Autodesk Inventor part; units mm, degrees
ref_plane "YZ Plane" through (0, 0, 0) normal (1, 0, 0) x (0, 1, 0)
ref_plane "XZ Plane" through (0, 0, 0) normal (0, 1, 0) x (-1, 0, 0)
ref_plane "XY Plane" through (0, 0, 0) normal (0, 0, 1) x (1, 0, 0)
sketch "Sketch1" plane through (0, 0, 0) normal (0, 0, 1) x (1, 0, 0)
  circle A0 centre (0, 0) radius 2
  circle A1 centre (0, 0) radius 8
  dimension "d0" = 4
  dimension "d1" = 16
extrude "Extrusion1" add sketch "Sketch1" along normal blind 6
sketch "Sketch2" plane through (0, 0, 6) normal (0, 0, 1) x (1, 0, 0)
  circle A0 centre (0, 0) radius 5
  circle A1 centre (0, 0) radius 15
  dimension "d4" = 10
  dimension "d5" = 30
extrude "Extrusion2" add sketch "Sketch2" along normal blind 5
sketch "Sketch5" plane through (0, 0, 6) normal (0, 0, -1) x (-1, 0, 0)
  circle A0 centre (0, 12.5) radius 1.4
  circle A1 centre (-12.5, 0) radius 1.4
  circle A2 centre (0, -12.5) radius 1.4
  circle A3 centre (12.5, 0) radius 1.4
  point P0 (0, 0)
  dimension "d24" = 12.5
  dimension "d25" = 2.8
  dimension "d28" = 360
extrude "Extrusion5" cut sketch "Sketch5" against normal blind 10 contours A0 | A1 | A3
sketch "Sketch6" plane through (0, 0, 11) normal (0, 0, 1) x (1, 0, 0)
  circle A0 centre (0, -12.5) radius 1.4
  point P0 (0, 0)
  dimension "d42" = 2.8
  dimension "d43" = 12.5
extrude "Extrusion6" cut sketch "Sketch6" against normal blind 10
sketch "Sketch9" plane through (0, 0, 0) normal (0, 0, -1) x (-1, 0, 0)
  line L0 (1.5, 2.0687) -> (1.5, -2.0687)
  circle A0 centre (0, 0) radius 2
  point P0 (1.5, 1.3229)
  point P1 (1.5, -1.3229)
  dimension "d46" = 4
  dimension "d47" = 1.5
extrude "Extrusion7" add sketch "Sketch9" against normal blind 6 contours A0 L0 picked at (1.7382, -0.2911)
sketch "Sketch11" plane through (0, 0, 0) normal (1, 0, 0) x (0, 1, 0)
  circle A0 centre (0, 3) radius 1
  line L0 (8, 0) -> (-8, 0)
  point P0 (0, 0)
  dimension "d50" = 2
  dimension "d51" = 3
extrude "Extrusion8" cut sketch "Sketch11" against normal blind 10
sketch "Sketch12" plane through (0, 0, 6) normal (0, 0, -1) x (-1, 0, 0)
  point P0 (0, 0)
sketch "Sketch13" plane through (0, 0, 6) normal (0, 0, -1) x (-1, 0, 0)
  point P0 (0, 0)
properties part number "motor dişlisi"
Work out the finished part from the listing and answer in its coordinate system (mm). A direction names the side the tool comes from. Coordinates: 2 decimals unless noted, no trailing zeros. Loops run counter-clockwise (first coordinate to the right, second up) from the corner with the lowest first, then second, coordinate; pieces in that order, holes last. Notation, with made-up numbers: (44, 21.5) -> (49, 21.5) arc R20 ccw to (49, 31.5) -> close; hole circle Ø6 at (43, 17). An arc over 180 degrees is marked (long way). Answer as CSV lines item,"result".
1) Straight lines are drawn through the part: probe 1 along Y at (x, z) = (0, 9); probe 2 along Y at (x, z) = (0, 3.85); probe 3 along X at (y, z) = (-0.5, 7.25). For each, find the intervals that lie inside material, in ascending order.
A:
probe 1,"y = -15 to -13.9, -11.1 to -5, 5 to 11.1, 13.9 to 15"
probe 2,"y = -8 to -2, 2 to 8"
probe 3,"x = -14.99 to -13.81, -11.19 to -4.97, 4.97 to 11.19, 13.81 to 14.99"
2) For a pull along X with two mould halves and no side action, classify faces 4 (the face through (-0.75, 13.68, 8.46)), 5 (the face through (7.39, 3.06, 2.96)), 6 (the face through (2, 0, 3)), 7 (the face through (-5, 0, 4)) as released by +X, released by -X, zero draft, split by the parting line, or undercut.
A:
face 4,"undercut"
face 5,"split by the parting line"
face 6,"undercut"
face 7,"zero draft"
3) The part is cut by section A-A (y = 0). Give the vertices of the cut face in (x, z), and give its area (3 significant figures).
A:
outline,"(-15, 6) -> (-13.9, 6) -> (-13.9, 11) -> (-15, 11) -> close; (-11.1, 6) -> (-8, 6) -> (-8, 4) -> (-1.5, 4) -> (-1.5, 6) -> (-5, 6) -> (-5, 11) -> (-11.1, 11) -> close; (-8, 0) -> (-1.5, 0) -> (-1.5, 2) -> (-8, 2) -> close; (2, 0) -> (8, 0) -> (8, 6) -> (11.1, 6) -> (11.1, 11) -> (5, 11) -> (5, 6) -> (2, 6) -> close; (13.9, 6) -> (15, 6) -> (15, 11) -> (13.9, 11) -> close"
area,"134 mm²"
4) The part is cut by section D-D (z = 0.5). Give the vertices of the cut face in (x, y), and give its area (3 significant figures).
A:
outline,"circle Ø16 at (0, 0); hole (-1.5, -1.32) arc R2 ccw (long way) to (-1.5, 1.32) -> close"
area,"189 mm²"
5) Flat-ended cylindrical pins translate along their axes: pin 1 (4.5 mm diameter, centred on x = -12.5, y = 0, fed in from -Z); pin 2 (1.2 mm diameter, centred on y = 0, z = 3, fed in from +X); pin 3 (2 mm diameter, centred on x = 4.5, z = 1.5, fed in from -Y). Find the tip coordinate at first contact, or state that the pin passes through.
A:
pin 1,"stops at z = 6"
pin 2,"stops at x = 8"
pin 3,"stops at y = -7.19"
6) For faces 1 (the face through (-1.5, 1, 2)), 2 (the face through (-1.08, 4.88, 8.46)), 3 (the face through (6, -6, 6)), determine the directions among +Z, -Z, +X, -X, +Y, -Y from which every point of the face is accessible in a straight line to the end or side of a thin tool.
A:
face 1,"+Z, -Z"
face 2,"+Z"
face 3,"-Z"
7) The part is cut by section B-B (x = 12.5). Give the vertices of the cut face in (y, z).
A:
outline,"(-8.29, 6) -> (-1.4, 6) -> (-1.4, 11) -> (-8.29, 11) -> close; (1.4, 6) -> (8.29, 6) -> (8.29, 11) -> (1.4, 11) -> close"
8) The part is cut by section C-C (z = 7.75). Give the vertices of the cut face in (x, y), and give its area (3 significant figures).
A:
outline,"circle Ø30 at (0, 0); hole circle Ø2.8 at (-12.5, 0); hole circle Ø10 at (0, 0); hole circle Ø2.8 at (0, -12.5); hole circle Ø2.8 at (0, 12.5); hole circle Ø2.8 at (12.5, 0)"
area,"604 mm²"
